The listing builds one solid part. Answer for the finished solid, in the listing's coordinates (mm). Give positions to 0.01 mm unless a question says otherwise; leave off trailing zeros. Loops run counter-clockwise (first coordinate to the right, second up) from the corner with the lowest first, then second, coordinate; pieces in that order, holes last. Notation, with made-up numbers: M 31,60 L 63,60 A16 ccw 63,77 Z; hole C -13,40 d3. An arc over 180 degrees is marked long. One line per item, written item: value. Start each with the question number.
Q1. A cutting plane is placed at B-B, the plane y = 0.5. State how many separate pieces and enclosed holes the cut face has, and give its area (3 significant figures).
Q2. A cutting plane is placed at A-A, the plane z = 51. Determine the outline of the cut face in (x, y) (3 decimals).
Q3. Consider L1, parallel to X at y = 2.2, z = -242.5; L2, parallel to X at y = 0.55, z = -249.5; L3, parallel to X at y = 1.05, z = -223. Determine where each line is inside the solid, lowest interval first.
Q4. Flat-ended cylindrical pins translate along their axes: pin 1 (10 mm diameter, centred on x = 12, z = -108, fed in from -Y); pin 2 (1.5 mm diameter, centred on y = 2, z = -111.5, fed in from +X); pin 3 (2 mm diameter, centred on x = -20.89, z = 242.5, fed in from +Y); pin 4 (1 mm diameter, centred on x = 19.5, y = 2, fed in from +Z). Find the tip coordinate at first contact, or state that the pin passes through.
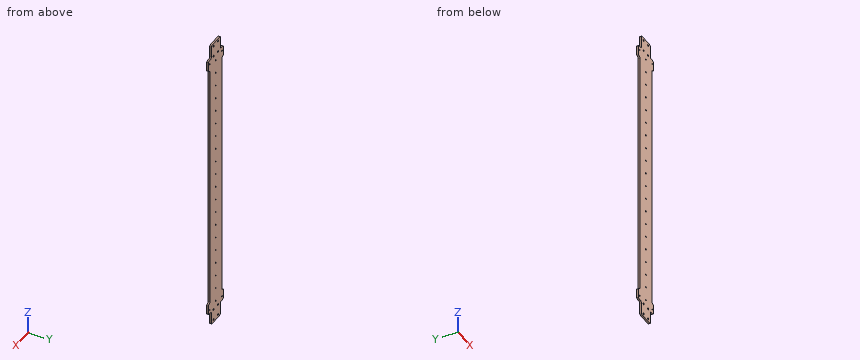
from build123d import *

# Parameters (mm, degrees)
BOSS_EXTRUDE1_DEPTH         = 3.175
FILLET1_R                   = 3.175
M3_CLEARANCE_HOLE1_D        = 3.4
FILLET2_R                   = 2
TAP_DRILL_FOR_M3X0_5_TAP1_D = 2.5
LPATTERN1_COUNT             = 10
LPATTERN1_PITCH             = 25
TAP_DRILL_FOR_M3X0_5_TAP2_D = 2.5
MIRROR1_COPY_1_D            = 2.5
MIRROR1_COPY_2_D            = 2.5
MIRROR1_COPY_3_D            = 2.5
MIRROR1_COPY_4_D            = 2.5
MIRROR1_COPY_5_D            = 2.5
MIRROR1_COPY_6_D            = 2.5
MIRROR1_COPY_7_D            = 2.5
MIRROR1_COPY_8_D            = 2.5
MIRROR1_COPY_9_D            = 2.5
FILLET1_OF_MIRROR1_R        = 3.175
FILLET2_OF_MIRROR1_R        = 2


with BuildPart() as part:
    # Sketch2 → Boss-Extrude1 (new body)
    with BuildSketch(Plane(origin=(0, 0, 0), x_dir=(1, 0, 0), z_dir=(0, 1, 0))):
        Polygon((-20, 0), (20, 0), (20, 230), (25, 230), (25, 250), (15, 250), (15, 275), (-15, 275), (-15, 250), (-25, 250), (-25, 230), (-20, 230), align=None)
    boss_extrude1 = extrude(amount=BOSS_EXTRUDE1_DEPTH)

    # Fillet1
    fillet1_edges = [part.edges().sort_by_distance(p)[0] for p in [
        (-20, 1.5875, -230),
        (-15, 1.5875, -250),
        (15, 1.5875, -250),
        (20, 1.5875, -230),
    ]]
    fillet(fillet1_edges, radius=FILLET1_R)

    # M3 Clearance Hole1 (through all)
    with Locations(Plane(origin=(-7.381007447, 3.175, -270), x_dir=(0, 0, 1), z_dir=(0, 1, 0))):
        with Locations((0, 0), (20, 0), (0, 15), (20, 15)):
            m3_clearance_hole1 = Hole(M3_CLEARANCE_HOLE1_D / 2)

    # Fillet2
    fillet2_edges = [part.edges().sort_by_distance(p)[0] for p in [
        (-25, 1.5875, -250),
        (15, 1.5875, -275),
        (-15, 1.5875, -275),
        (-25, 1.5875, -230),
        (25, 1.5875, -230),
        (25, 1.5875, -250),
    ]]
    fillet(fillet2_edges, radius=FILLET2_R)

    # Tap Drill for M3x0.5 Tap1 (through all)
    with Locations(Plane(origin=(0.113042925, 3.175, -237.5), x_dir=(0, 0, 1), z_dir=(0, 1, 0))):
        with Locations((0, 0)):
            tap_drill_for_m3x0_5_tap1 = Hole(TAP_DRILL_FOR_M3X0_5_TAP1_D / 2)

    # LPattern1: Tap Drill for M3x0.5 Tap1 ×10
    with Locations(*[(0, 0, i * LPATTERN1_PITCH) for i in range(1, LPATTERN1_COUNT)]):
        add(tap_drill_for_m3x0_5_tap1, mode=Mode.SUBTRACT)

    # Tap Drill for M3x0.5 Tap2 (through all)
    with Locations(Plane(origin=(-20.886041747, 3.175, -242.5), x_dir=(0, 0, 1), z_dir=(0, 1, 0))):
        with Locations((0, 0), (0, 42)):
            tap_drill_for_m3x0_5_tap2 = Hole(TAP_DRILL_FOR_M3X0_5_TAP2_D / 2)

    # Mirror1: Boss-Extrude1, M3 Clearance Hole1, Tap Drill for M3x0.5 Tap1, Tap Drill for M3x0.5 Tap2 across plane
    add(boss_extrude1.mirror(Plane.XY))
    add(m3_clearance_hole1.mirror(Plane.XY), mode=Mode.SUBTRACT)
    add(tap_drill_for_m3x0_5_tap1.mirror(Plane.XY), mode=Mode.SUBTRACT)
    add(tap_drill_for_m3x0_5_tap2.mirror(Plane.XY), mode=Mode.SUBTRACT)

    # Mirror1 copy 1 (through all)
    with Locations(Plane(origin=(0.113042925, 3.175, 212.5), x_dir=(0, 0, -1), z_dir=(0, 1, 0))):
        with Locations((0, 0)):
            Hole(MIRROR1_COPY_1_D / 2)

    # Mirror1 copy 2 (through all)
    with Locations(Plane(origin=(0.113042925, 3.175, 187.5), x_dir=(0, 0, -1), z_dir=(0, 1, 0))):
        with Locations((0, 0)):
            Hole(MIRROR1_COPY_2_D / 2)

    # Mirror1 copy 3 (through all)
    with Locations(Plane(origin=(0.113042925, 3.175, 162.5), x_dir=(0, 0, -1), z_dir=(0, 1, 0))):
        with Locations((0, 0)):
            Hole(MIRROR1_COPY_3_D / 2)

    # Mirror1 copy 4 (through all)
    with Locations(Plane(origin=(0.113042925, 3.175, 137.5), x_dir=(0, 0, -1), z_dir=(0, 1, 0))):
        with Locations((0, 0)):
            Hole(MIRROR1_COPY_4_D / 2)

    # Mirror1 copy 5 (through all)
    with Locations(Plane(origin=(0.113042925, 3.175, 112.5), x_dir=(0, 0, -1), z_dir=(0, 1, 0))):
        with Locations((0, 0)):
            Hole(MIRROR1_COPY_5_D / 2)

    # Mirror1 copy 6 (through all)
    with Locations(Plane(origin=(0.113042925, 3.175, 87.5), x_dir=(0, 0, -1), z_dir=(0, 1, 0))):
        with Locations((0, 0)):
            Hole(MIRROR1_COPY_6_D / 2)

    # Mirror1 copy 7 (through all)
    with Locations(Plane(origin=(0.113042925, 3.175, 62.5), x_dir=(0, 0, -1), z_dir=(0, 1, 0))):
        with Locations((0, 0)):
            Hole(MIRROR1_COPY_7_D / 2)

    # Mirror1 copy 8 (through all)
    with Locations(Plane(origin=(0.113042925, 3.175, 37.5), x_dir=(0, 0, -1), z_dir=(0, 1, 0))):
        with Locations((0, 0)):
            Hole(MIRROR1_COPY_8_D / 2)

    # Mirror1 copy 9 (through all)
    with Locations(Plane(origin=(0.113042925, 3.175, 12.5), x_dir=(0, 0, -1), z_dir=(0, 1, 0))):
        with Locations((0, 0)):
            Hole(MIRROR1_COPY_9_D / 2)

    # Fillet1 of Mirror1
    fillet1_of_mirror1_edges = [part.edges().sort_by_distance(p)[0] for p in [
        (-20, 1.5875, 230),
        (-15, 1.5875, 250),
        (15, 1.5875, 250),
        (20, 1.5875, 230),
    ]]
    fillet(fillet1_of_mirror1_edges, radius=FILLET1_OF_MIRROR1_R)

    # Fillet2 of Mirror1
    fillet2_of_mirror1_edges = [part.edges().sort_by_distance(p)[0] for p in [
        (-25, 1.5875, 250),
        (15, 1.5875, 275),
        (-15, 1.5875, 275),
        (-25, 1.5875, 230),
        (25, 1.5875, 230),
        (25, 1.5875, 250),
    ]]
    fillet(fillet2_of_mirror1_edges, radius=FILLET2_OF_MIRROR1_R)


solid = part.part
Answer block:
1. separate pieces: 1
1. enclosed holes: 32
1. area: 21,700 mm^2
2. outline: M -20,0 L 20,0 L 20,3.175 L -20,3.175 Z
3. L1: -25 to -22.14, -19.64 to 19.86, 22.36 to 25
3. L2: -24.32 to -9.01, -5.76 to 5.99, 9.24 to 24.32
3. L3: -20 to 20
4. pin 1: y = 0
4. pin 2: x = 20
4. pin 3: through
4. pin 4: z = 250
